from build123d import *
from build123d.topology import SkipClean

# Parameters (mm, degrees)
SKETCH1_R           = 85.32472163
BOSS_EXTRUDE1_DEPTH = 40
BOSS_EXTRUDE6_DEPTH = 80
SKETCH7_R           = 50
CUT_EXTRUDE1_DEPTH  = 20
SKETCH8_R           = 15
CUT_EXTRUDE2_DEPTH  = 60


with BuildPart() as part:
    # Sketch1 → Boss-Extrude1 (new body)
    with BuildSketch(Plane(origin=(0, 0, 0), x_dir=(1, 0, 0), z_dir=(0, 1, 0))):
        with Locations(Location((0, 0, 0), (0, 0, 270))):
            Circle(SKETCH1_R)
    extrude(amount=BOSS_EXTRUDE1_DEPTH)

    # Sketch2 → Boss-Extrude6 (add)
    with SkipClean():  # the faces are left unmerged after this step: merging them gives an invalid solid
        with BuildSketch(Plane(origin=(0, 40, 0), x_dir=(1, 0, 0), z_dir=(0, 1, 0))):
            with BuildLine():
                Line((8.607565416, -5.090168722), (73.443812301, -43.431722922))
                ThreePointArc((73.443812301, -43.431722922), (82.182232136, -22.943165483), (85.320068664, -0.89106923))
                Line((85.320068664, -0.89106923), (10, 0))
                ThreePointArc((10, 0), (9.645611804, -2.638592981), (8.607565416, -5.090168722))
            make_face()
            with BuildLine():
                Line((-5.02968533, -8.643047234), (-42.915650066, -73.746559925))
                ThreePointArc((-42.915650066, -73.746559925), (-22.366320531, -82.341094401), (-0.292763215, -85.324219369))
                Line((-0.292763215, -85.324219369), (-0.034311652, -9.999941135))
                ThreePointArc((-0.034311652, -9.999941135), (-2.621317726, -9.650320895), (-5.02968533, -8.643047234))
            make_face()
            with BuildLine():
                Line((-10, 0), (-85.32472163, 0))
                ThreePointArc((-85.32472163, 0), (-82.417352244, 22.083662976), (-73.893376503, 42.662360815))
                Line((-73.893376503, 42.662360815), (-8.660254038, 5))
                ThreePointArc((-8.660254038, 5), (-9.659258263, 2.588190451), (-10, 0))
            make_face()
            with BuildLine():
                Line((0, 10), (0, 85.32472163))
                ThreePointArc((0, 85.32472163), (22.083662976, 82.417352244), (42.662360815, 73.893376503))
                Line((42.662360815, 73.893376503), (5, 8.660254038))
                ThreePointArc((5, 8.660254038), (2.588190451, 9.659258263), (0, 10))
            make_face()
        extrude(amount=BOSS_EXTRUDE6_DEPTH)

    # Sketch6 → Cut-Revolve1 (revolve, cut)
    with SkipClean():  # the faces are left unmerged after this step: merging them gives an invalid solid
        with BuildSketch(Plane(origin=(0, 0, 0), x_dir=(0.5000000000000012, 0, -0.866025403784438), z_dir=(0.8660254037844379, 0, 0.5000000000000011)), mode=Mode.PRIVATE) as cut_revolve1_sk:
            with BuildLine():
                Line((85.32472163, 120), (0, 120))
                Line((0, 120), (0, 34.67527837))
                ThreePointArc((0, 34.67527837), (60.333689268, 59.666310732), (85.32472163, 120))
            make_face()
        revolve(cut_revolve1_sk.sketch.rotate(Axis((0, 120, 0), (0, -1, 0)), 330), axis=Axis((0, 120, 0), (0, -1, 0)), mode=Mode.SUBTRACT)

    # Sketch7 → Cut-Extrude1 (cut)
    with SkipClean():  # the faces are left unmerged after this step: merging them gives an invalid solid
        with BuildSketch(Plane.XZ):
            with Locations(Location((0, 0, 0), (0, 0, 270))):
                Circle(SKETCH7_R)
        extrude(amount=-CUT_EXTRUDE1_DEPTH, mode=Mode.SUBTRACT)

    # Sketch8 → Cut-Extrude2 (cut)
    with SkipClean():  # the faces are left unmerged after this step: merging them gives an invalid solid
        with BuildSketch(Plane.XZ.offset(-20)):
            with Locations(Location((0, 0, 0), (0, 0, 270))):
                Circle(SKETCH8_R)
        extrude(amount=-CUT_EXTRUDE2_DEPTH, mode=Mode.SUBTRACT)


solid = part.part
Can you work these out from the model? Positions are in its coordinate system, mm. A direction names the side the tool comes from. Round coordinates to 2 decimals unless told otherwise and drop trailing zeros. Write each loop counter-clockwise with the first axis right and the second up, starting at its lowest first coordinate (ties: lowest second). Pieces come first, ordered by that corner, then holes. Notation, with made-up numbers: (60, -3) -> (115, -3) arc R22 ccw to (115, 36) -> close; hole circle Ø1 at (55.25, -4.5). An arc over 180 degrees is marked (long way). Use one line per item in the form item = value. Start each with the question number.
Q1. Imagine slicing it at B-B (y = 99). Please give me the cut outline in (x, z).
Q2. Imagine slicing it at D-D (x = -67). Please give me the cut outline in (y, z).
Q3. We'd pull the mould along Z, two halves only. Please class faces 1 (the face through (51, 40, -29)), 2 (the face through (29, 40, 50)), 3 (the face through (60.03, 59.07, 35.5)): +Z half, -Z half, draft (parallel to the pull), parting line (faces both ways), or undercut.
Q4. I'm going to push flat-ended pins straight in: P1, Ø1.5, axis at y = 35.5, z = 33, coming from the +X side; P2, Ø12, axis at x = -10.5, y = 49, coming from the +Z side; P3, Ø21, axis at x = 51, z = 54.5, coming from the +Y side; P4, Ø24, axis at x = 0, z = 0, coming from the +Y side. Where does each tip first touch, or does it pass through?
Q5. If I drill on probe 1 along X at (y, z) = (12.25, 0); probe 2 along X at (y, z) = (30.5, 0); probe 3 along Y at (x, z) = (67.5, -12), over which ranges is the centre line in solid material (lowest first)? Write a range as [from, to].
Q6. Imagine slicing it at A-A (z = -6.5). Please give me the cut outline in (x, y), then the cut area to 3 significant figures.
Q7. Which directions (+Z, -Z, +X, -X, +Y, -Y) give clear straight access to the entire face, cutting with the end or side of a thin tool? Please do faces 4 (the face through (12, 20, -10)), 5 (the face through (-28, 40, -51)), 6 (the face through (-50, 40, 28)), 7 (the face through (-37, 0, 37)), 8 (the face through (36.028, 59.073, -62.403)).
Q8. Imagine slicing it at C-C (z = 56.5). Please give me the cut outline in (x, y).
Worked out:
q1.outline = (-85.32, 0) arc R85.32 ccw to (-73.89, -42.66) -> (-71.62, -41.35) arc R82.7 cw to (-82.7, 0) -> close; (-42.92, 73.75) -> (-41.6, 71.48) arc R82.7 cw to (-0.28, 82.7) -> (-0.29, 85.32) arc R85.32 ccw to start; (0, -85.32) arc R85.32 ccw to (42.66, -73.89) -> (41.35, -71.62) arc R82.7 cw to (0, -82.7) -> close; (71.18, 42.1) arc R82.7 cw to (82.7, 0.86) -> (85.32, 0.89) arc R85.32 ccw to (73.44, 43.43) -> close
q2.outline = (0, -52.83) -> (40, -52.83) -> (40, -38.68) -> (84.01, -38.68) arc R52.83 cw to (67.17, 0) -> (40, 0) -> (40, 52.83) -> (0, 52.83) -> close
q3.face_1 = undercut
q3.face_2 = draft
q3.face_3 = +Z half
q4.P1 = 79
q4.P2 = 85.21
q4.P3 = 40
q4.P4 = through
q5.probe_1 = [-85.32, -50], [50, 85.32]
q5.probe_2 = [-85.32, -15], [15, 85.32]
q5.probe_3 = [0, 40]
q6.outline = (-85.08, 0) -> (-49.58, 0) -> (-49.58, 20) -> (-13.52, 20) -> (-13.52, 36) arc R85.08 cw to (-85.08, 120) -> close; (13.52, 20) -> (49.58, 20) -> (49.58, 0) -> (85.08, 0) -> (85.08, 40) -> (28.95, 40) arc R85.08 cw to (13.52, 36) -> close
q6.area = 5,430 mm^2
q7.face_4 = -Y
q7.face_5 = -Z, +Y
q7.face_6 = -X, +Y
q7.face_7 = +Z, -Z, +X, -X, -Y
q7.face_8 = +X, +Y
q8.outline = (-63.94, 0) -> (63.94, 0) -> (63.94, 40) -> (-0.19, 40) -> (-0.19, 56.06) arc R63.94 cw to (-32.88, 65.16) -> (-32.88, 40) -> (-63.94, 40) -> close
